Model file for the job. Use its own axes, mm. Coordinates: 2 decimals unless noted, no trailing zeros.
Q1. Pin check, flat tips, straight feed: P1, Ø3, axis at y = 150, z = -15.5, coming from the -X side (1 decimal); P2, Ø6, axis at y = -22.5, z = 50, coming from the +X side. Stop position of each tip, or through.
Q2. Drill centre lines: probe 1 along Z at (x, y) = (4, 74); probe 2 along Z at (x, y) = (1.9, -224); probe 3 along Y at (x, z) = (3.6, 0). Where is each one in solid material? Low to high.
Q3. Pull direction Z, two halves, no side cores. Call faces 1 (the cylindrical face through (2.535, 157.436, 0.976)), 2 (the flat face through (0, 4, 2)): released by +Z, released by -Z, zero draft, split by the parting line, or undercut.
Autodesk Inventor part; units mm, degrees
ref_plane "YZ Plane" through (0, 0, 0) normal (1, 0, 0) x (0, 1, 0)
ref_plane "XZ Plane" through (0, 0, 0) normal (0, 1, 0) x (-1, 0, 0)
ref_plane "XY Plane" through (0, 0, 0) normal (0, 0, 1) x (1, 0, 0)
sketch "草图1" plane through (0, 0, 0) normal (1, 0, 0) x (0, 1, 0)
  line L0 (250, 140) -> (-250, 140)
  line L1 (-250, 140) -> (-250, -150)
  line L2 (-250, -150) -> (250, -150)
  line L3 (250, -150) -> (250, 140)
  point P0 (0, 0)
  dimension "d0" = 500
  dimension "d1" = 290
extrude "拉伸1" add sketch "草图1" along normal blind 5
sketch "草图2" plane through (5, 0, 0) normal (1, 0, 0) x (0, 0, -1)
  circle A0 centre (85.5, -224) radius 1.8
  point P0 (0, 0)
  dimension "d4" = 3.6
extrude "拉伸2" cut sketch "草图2" against normal through all
sketch "草图3" plane through (5, 0, 0) normal (1, 0, 0) x (0, 0, -1)
  circle A0 centre (-85.5, -224) radius 1.8
  point P0 (0, 0)
  dimension "d7" = 3.6
extrude "拉伸3" cut sketch "草图3" against normal through all
sketch "草图4" plane through (0, 0, 0) normal (-1, 0, 0) x (0, 0, 1)
  circle A0 centre (54.5, -224) radius 1.8
  point P0 (0, 0)
  dimension "d10" = 3.6
extrude "拉伸4" cut sketch "草图4" against normal through all
sketch "草图5" plane through (5, 0, 0) normal (1, 0, 0) x (0, 0, -1)
  circle A0 centre (54.5, -224) radius 1.8
  point P0 (0, 0)
  dimension "d13" = 3.6
extrude "拉伸5" cut sketch "草图5" against normal through all
sketch "草图8" plane through (5, 0, 0) normal (1, 0, 0) x (0, 0, -1)
  circle A0 centre (-119, 165.5) radius 1.8
  point P0 (0, 0)
  dimension "d22" = 3.6
extrude "拉伸8" cut sketch "草图8" against normal through all
sketch "草图9" plane through (0, 0, 0) normal (-1, 0, 0) x (0, 0, 1)
  circle A0 centre (119, 134.5) radius 1.8
  point P0 (0, 0)
  dimension "d25" = 3.6
extrude "拉伸9" cut sketch "草图9" against normal through all
sketch "草图10" plane through (5, 0, 0) normal (1, 0, 0) x (0, 0, -1)
  circle A0 centre (119, 134.5) radius 1.8
  point P0 (0, 0)
  dimension "d28" = 3.6
extrude "拉伸10" cut sketch "草图10" against normal through all
sketch "草图11" plane through (5, 0, 0) normal (1, 0, 0) x (0, 0, -1)
  circle A0 centre (119, 165.5) radius 1.8
  point P0 (0, 0)
  dimension "d31" = 3.6
extrude "拉伸11" cut sketch "草图11" against normal through all
sketch "草图12" plane through (5, 0, 0) normal (1, 0, 0) x (0, 0, -1)
  line L0 (145, -250) -> (150, -250)
  line L1 (150, -250) -> (150, 250)
  line L2 (150, 250) -> (145, 250)
  line L3 (145, 250) -> (145, -250)
  point P0 (0, 0)
  dimension "d34" = 5
  dimension "d35" = 500
extrude "拉伸12" cut sketch "草图12" against normal through all
sketch "草图13" plane through (5, 0, 0) normal (1, 0, 0) x (0, 0, -1)
  line L0 (-140, -250) -> (-145, -250)
  line L1 (-145, -250) -> (-145, 250)
  line L2 (-145, 250) -> (-140, 250)
  line L3 (-140, 250) -> (-140, -250)
  point P0 (0, 0)
  dimension "d38" = 5
  dimension "d39" = 500
extrude "拉伸13" add sketch "草图13" against normal blind 5
sketch "草图14" plane through (5, 0, 0) normal (1, 0, 0) x (0, 0, -1)
  circle A0 centre (0, 0) radius 1.8
  dimension "d42" = 3.6
extrude "拉伸14" cut sketch "草图14" against normal through all
sketch "草图15" plane through (5, 0, 0) normal (1, 0, 0) x (0, 0, -1)
  circle A0 centre (48.4, 0) radius 1.8
  point P0 (0, 0)
  dimension "d45" = 3.6
extrude "拉伸15" cut sketch "草图15" against normal through all
sketch "草图16" plane through (5, 0, 0) normal (1, 0, 0) x (0, 0, -1)
  circle A0 centre (0, -74.8) radius 1.8
  point P0 (0, 0)
  dimension "d48" = 3.6
extrude "拉伸16" cut sketch "草图16" against normal through all
sketch "草图17" plane through (5, 0, 0) normal (1, 0, 0) x (0, 0, -1)
  circle A0 centre (48.4, -81.8) radius 1.8
  point P0 (0, 0)
  dimension "d51" = 3.6
extrude "拉伸17" cut sketch "草图17" against normal through all
sketch "草图18" plane through (5, 0, 0) normal (1, 0, 0) x (0, 0, -1)
  circle A0 centre (0, 37) radius 1.8
  point P0 (0, 0)
  dimension "d54" = 3.6
extrude "拉伸18" cut sketch "草图18" against normal through all
sketch "草图19" plane through (5, 0, 0) normal (1, 0, 0) x (0, 0, -1)
  circle A0 centre (37, 74) radius 1.8
  point P0 (0, 0)
  dimension "d57" = 3.6
extrude "拉伸19" cut sketch "草图19" against normal through all
sketch "草图20" plane through (5, 0, 0) normal (1, 0, 0) x (0, 0, -1)
  circle A0 centre (0, 74) radius 1.8
  point P0 (0, 0)
  dimension "d60" = 3.6
extrude "拉伸20" cut sketch "草图20" against normal through all
sketch "草图21" plane through (5, 0, 0) normal (1, 0, 0) x (0, 0, -1)
  circle A0 centre (37, 37) radius 1.8
  point P0 (0, 0)
  dimension "d63" = 3.6
extrude "拉伸21" cut sketch "草图21" against normal through all
sketch "草图22" plane through (5, 0, 0) normal (1, 0, 0) x (0, 0, -1)
  circle A0 centre (-50, -22.5) radius 2.5
  point P0 (0, 0)
  dimension "d66" = 5
extrude "拉伸22" cut sketch "草图22" against normal through all
sketch "草图23" plane through (5, 0, 0) normal (1, 0, 0) x (0, 0, -1)
  circle A0 centre (-50, 22.5) radius 2.5
  point P0 (0, 0)
  dimension "d69" = 5
extrude "拉伸23" cut sketch "草图23" against normal through all
sketch "草图24" plane through (5, 0, 0) normal (1, 0, 0) x (0, 0, -1)
  circle A0 centre (-100, -22.5) radius 2.5
  point P0 (0, 0)
  dimension "d72" = 5
extrude "拉伸24" cut sketch "草图24" against normal through all
sketch "草图25" plane through (5, 0, 0) normal (1, 0, 0) x (0, 0, -1)
  circle A0 centre (-100, 22.5) radius 2.5
  point P0 (0, 0)
  dimension "d75" = 5
extrude "拉伸25" cut sketch "草图25" against normal through all
sketch "草图26" plane through (5, 0, 0) normal (1, 0, 0) x (0, 0, -1)
  circle A0 centre (15.5, 150) radius 1.8
  point P0 (0, 0)
  dimension "d78" = 3.6
extrude "拉伸26" cut sketch "草图26" against normal through all
sketch "草图27" plane through (5, 0, 0) normal (1, 0, 0) x (0, 0, -1)
  circle A0 centre (-15.5, 150) radius 1.8
  point P0 (0, 0)
  dimension "d81" = 3.6
extrude "拉伸27" cut sketch "草图27" against normal through all
sketch "草图28" plane through (5, 0, 0) normal (1, 0, 0) x (0, 0, -1)
  circle A0 centre (0, 150) radius 7.5
  point P0 (0, 0)
  dimension "d84" = 15
extrude "拉伸28" cut sketch "草图28" against normal through all
equation "\"折弯半径\" = 厚度"
equation "\"折弯释压宽度\" = 厚度"
equation "\"折弯释压深度\" = 0.5 * 厚度"
equation "\"拐角释压尺寸\" = 4 * 厚度"
equation "\"最小余量\" = 2 * 厚度"
equation "\"过渡半径\" = 折弯半径"
equation "\"Jacobi半径尺寸\" = 折弯半径"
equation "\"间隙大小\" = 厚度"
properties part number "290mm板"
Answer sheet:
1. P1: passes through
1. P2: stops at x = 5
2. probe 1: z = -145 to -38.8, -35.2 to -1.8, 1.8 to 145
2. probe 2: z = -145 to -87.3, -83.7 to -56.3, -52.7 to 52.7, 56.3 to 83.7, 87.3 to 145
2. probe 3: y = -250 to -76.6, -73 to -1.8, 1.8 to 35.2, 38.8 to 72.2, 75.8 to 142.5, 157.5 to 250
3. face 1: undercut
3. face 2: zero draft
